Here's how the part is built. I have some questions about the finished solid (model axes, mm). Round coordinates to 2 decimals unless told otherwise and drop trailing zeros. Write each loop counter-clockwise with the first axis right and the second up, starting at its lowest first coordinate (ties: lowest second). Pieces come first, ordered by that corner, then holes. Notation, with made-up numbers: (77, 39) -> (130, 39) arc R27 cw to (130, 65) -> close; hole circle Ø8 at (22, 53). An arc over 180 degrees is marked (long way). Put each result on its own line as item: value. Start each with the question number.
1. Suppose I cut it at B-B (z = 2.25). Please give me the cut outline in (x, y).
2. Suppose I cut it at D-D (x = 41). Count the separate pieces of the cut face and the enclosed holes in it, then the cut area to 3 significant figures.
3. Suppose I cut it at A-A (y = 0). Please give me the cut outline in (x, z), then the cut area to 3 significant figures.
4. I need wall thicknesses on probe 1 along X at (y, z) = (-41, 4.5); probe 2 along X at (y, z) = (-26, 6). Which ranges of each line are inside material? Lowest first, please. Write a range as from..to.
```python
from build123d import *

# Parameters (mm, degrees)
SKETCH_W           = 105
SKETCH_H           = 105
PAD_DEPTH          = 7
SKETCH002_R        = 1.7
POCKET_DEPTH       = 9
POLARPATTERN_COUNT = 4
SKETCH001_R        = 46.59
POCKET001_DEPTH    = 8
FILLET_R           = 2
FILLET001_R        = 1


with BuildPart() as part:
    # Sketch → Pad (new body)
    with BuildSketch(Plane.XY):
        Rectangle(SKETCH_W, SKETCH_H)
    extrude(amount=PAD_DEPTH)

    # Sketch002 (on Face6 of Pad) → Pocket (cut)
    with BuildSketch(Plane.XY.offset(7)):
        with Locations((-41, 41)):
            Circle(SKETCH002_R)
    pocket = extrude(amount=-POCKET_DEPTH, mode=Mode.SUBTRACT)

    # PolarPattern: Pocket ×4 about axis
    polarpattern_axis = Axis((0, 0, 7), (0, 0, 1))
    for i in range(1, POLARPATTERN_COUNT):
        add(pocket.rotate(polarpattern_axis, i * 360 / POLARPATTERN_COUNT), mode=Mode.SUBTRACT)

    # Sketch001 (on Face6 of Pad) → Pocket001 (cut)
    with BuildSketch(Plane.XY.offset(7)):
        Circle(SKETCH001_R)
    extrude(amount=-POCKET001_DEPTH, mode=Mode.SUBTRACT)

    # Fillet
    fillet_edges = [part.edges().sort_by_distance(p)[0] for p in [
        (-46.59, 0, 7),
    ]]
    fillet(fillet_edges, radius=FILLET_R)

    # Fillet001
    fillet001_edges = [part.edges().sort_by_distance(p)[0] for p in [
        (52.5, 0, 0),
        (-52.5, 0, 0),
        (0, -52.5, 0),
        (0, 52.5, 0),
    ]]
    fillet(fillet001_edges, radius=FILLET001_R)


solid = part.part
```
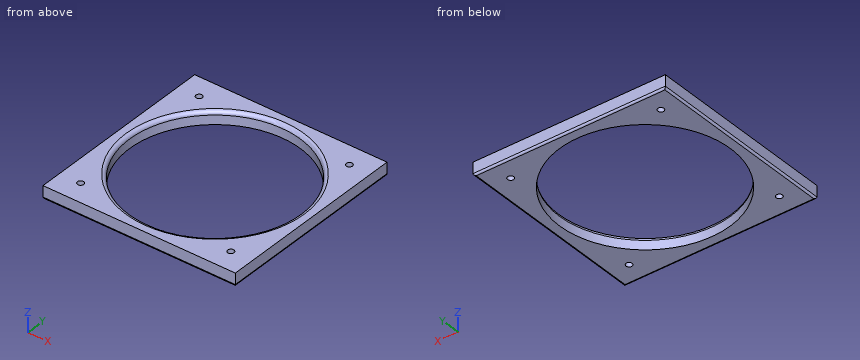
Verdict:
1. outline: (-52.5, -52.5) -> (52.5, -52.5) -> (52.5, 52.5) -> (-52.5, 52.5) -> close; hole circle Ø93.18 at (0, 0); hole circle Ø3.4 at (-41, -41); hole circle Ø3.4 at (-41, 41); hole circle Ø3.4 at (41, -41); hole circle Ø3.4 at (41, 41)
2. separate pieces: 4
2. enclosed holes: 0
2. area: 374 mm^2
3. outline: (-52.5, 1) arc R1 ccw to (-51.5, 0) -> (-46.59, 0) -> (-46.59, 5) arc R2 ccw to (-48.59, 7) -> (-52.5, 7) -> close; (46.59, 0) -> (51.5, 0) arc R1 ccw to (52.5, 1) -> (52.5, 7) -> (48.59, 7) arc R2 ccw to (46.59, 5) -> close
3. area: 80.6 mm^2
4. probe 1: x = -52.5..-42.7, -39.3..-22.13, 22.13..39.3, 42.7..52.5
4. probe 2: x = -52.5..-38.98, 38.98..52.5
